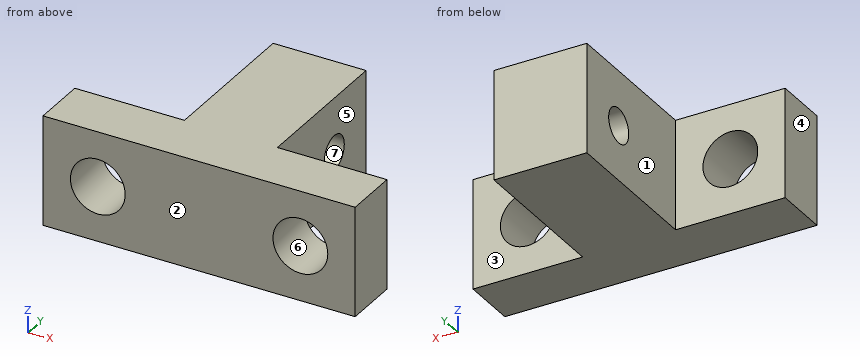
```python
from build123d import *

# Parameters (mm, degrees)
SKETCH1_W           = 10.7696
SKETCH1_H           = 17.699
BOSS_EXTRUDE1_DEPTH = 12.7
SKETCH5_R           = 2
CUT_EXTRUDE2_DEPTH  = 24.4696
SKETCH6_R           = 3.175
CUT_EXTRUDE3_DEPTH  = 7.35


with BuildPart() as part:
    # Sketch1 → Boss-Extrude1 (new body)
    with BuildSketch(Plane.XY):
        Polygon((18.0848, -8.8495), (5.3848, -8.8495), (-5.3848, -8.8495), (-18.0848, -8.8495), (-18.0848, -15.1995), (18.0848, -15.1995), align=None)
        Rectangle(SKETCH1_W, SKETCH1_H)
    extrude(amount=BOSS_EXTRUDE1_DEPTH)

    # Sketch5 → Cut-Extrude2 (cut, through all)
    with BuildSketch(Plane(origin=(5.3848, 0, 0), x_dir=(0, 0, -1), z_dir=(1, 0, 0))):
        with Locations((-6.35, 2.4995)):
            Circle(SKETCH5_R)
    extrude(amount=-CUT_EXTRUDE2_DEPTH, mode=Mode.SUBTRACT)

    # Sketch6 → Cut-Extrude3 (cut, through all)
    with BuildSketch(Plane(origin=(0, -8.8495, 0), x_dir=(1, 0, 0), z_dir=(0, 1, 0))):
        with Locations((-11.7348, -6.35)):
            Circle(SKETCH6_R)
        with Locations((11.7348, -6.35)):
            Circle(SKETCH6_R)
    extrude(amount=-CUT_EXTRUDE3_DEPTH, mode=Mode.SUBTRACT)


solid = part.part
```
For this review, take the finished solid that the model builds, in its own axes (mm). Face numbers are marked on the shaded views. A direction names the side the tool comes from. Give positions to 0.01 mm unless a question says otherwise; leave off trailing zeros. Write each loop counter-clockwise with the first axis right and the second up, starting at its lowest first coordinate (ties: lowest second). Pieces come first, ordered by that corner, then holes. Notation, with made-up numbers: M 17.25,6 L 32.25,6 A17 cw 32.25,14 Z; hole C -8,78.5 d2. An arc over 180 degrees is marked long. One line per item, written item: value.
1) For P1, Ø4, axis at y = 2, z = 8, coming from the -X side; P2, Ø8, axis at x = 7.5, y = 0, coming from the +Z side; P3, Ø5.5, axis at x = -11.73, z = 6.35, coming from the +Y side, all flat-tipped, find the tip position at first contact; note any pin that passes through.
Results are:
P1: stops at x = -5.38
P2: stops at z = 12.7
P3: passes through
2) Take a section at A-A, the plane z = 6.35. Write out the cut boundary in (x, y), then the cut area to 3 significant figures.
Results are:
outline: M -18.08,-15.2 L -14.91,-15.2 L -14.91,-8.85 L -18.08,-8.85 Z; M -8.56,-15.2 L 8.56,-15.2 L 8.56,-8.85 L 5.38,-8.85 L 5.38,0.5 L -5.38,0.5 L -5.38,-8.85 L -8.56,-8.85 Z; M -5.38,4.5 L 5.38,4.5 L 5.38,8.85 L -5.38,8.85 Z; M 14.91,-15.2 L 18.08,-15.2 L 18.08,-8.85 L 14.91,-8.85 Z
area: 297 mm²
3) For the marked faces 1, 2 and 3, list the 3-axis set-ups (+Z, -Z, +X, -X, +Y, -Y) from which the entire face can be reached by the end or side of a thin tool; tool diameter is ignored.
Results are:
face 1: +Z, -Z, -X, +Y
face 2: +Z, -Z, +X, -X, -Y
face 3: +Z, -Z, +X, +Y
4) For line 1 (X direction, y = -12.5, z = 6.35); line 2 (Y direction, x = 1, z = 6.35); line 3 (X direction, y = 6, z = 10.75), list the stretches that pass through material, from the lowest coordinate up. Write a range as from..to.
Results are:
line 1: x = -18.08..-14.91, -8.56..8.56, 14.91..18.08
line 2: y = -15.2..0.5, 4.5..8.85
line 3: x = -5.38..5.38
5) Take a section at B-B, the plane y = 4. Write out the cut boundary in (x, z), then the cut area to 3 significant figures.
Results are:
outline: M -5.38,0 L 5.38,0 L 5.38,5.03 L -5.38,5.03 Z; M -5.38,7.67 L 5.38,7.67 L 5.38,12.7 L -5.38,12.7 Z
area: 108 mm²
6) Take a section at D-D, the plane x = -12. Write out the cut boundary in (y, z).
Results are:
outline: M -15.2,0 L -8.85,0 L -8.85,3.19 L -15.2,3.19 Z; M -15.2,9.51 L -8.85,9.51 L -8.85,12.7 L -15.2,12.7 Z
7) Take a section at C-C, the plane z = 12. Write out the cut boundary in (x, y).
Results are:
outline: M -18.08,-15.2 L 18.08,-15.2 L 18.08,-8.85 L 5.38,-8.85 L 5.38,8.85 L -5.38,8.85 L -5.38,-8.85 L -18.08,-8.85 Z
8) The part is to be moulded in two halves that separate along X. For the marked faces 4, 5, 6 and 7, say which applies: +X half, -X half, draft (parallel to the pull), parting line (faces both ways), or undercut.
Results are:
face 4: -X half
face 5: +X half
face 6: undercut
face 7: draft
